Could you check a few things on this model? Use its own coordinates, in mm. A direction names the side the tool comes from. Coordinates: 2 decimals unless noted, no trailing zeros. Write each loop counter-clockwise with the first axis right and the second up, starting at its lowest first coordinate (ties: lowest second). Pieces come first, ordered by that corner, then holes.
```python
from build123d import *

# Parameters (mm, degrees)
SKETCH1_R               = 14.2875
SKETCH1_R_2             = 9.525
BOSS_EXTRUDE1_DEPTH     = 3.175
F_10_CLEARANCE_HOLE2_D  = 4.9784
F_10_CLEARANCE_HOLE3_D  = 4.9784
F_1_4_CLEARANCE_HOLE1_D = 6.5278


with BuildPart() as part:
    # Sketch1 → Boss-Extrude1 (new body)
    with BuildSketch(Plane.XY.offset(-14.194599474)):
        with BuildLine():
            Line((-11.403602879, 461.040918113), (18.881283072, 509.506866808))
            Line((18.881283072, 509.506866808), (22.784668372, 515.753589084))
            Line((22.784668372, 515.753589084), (19.342339301, 522.227668471))
            Line((19.342339301, 522.227668471), (12.014457551, 522.48356374))
            Line((12.014457551, 522.48356374), (8.11107225, 516.236841464))
            Line((8.11107225, 516.236841464), (-23.846467356, 536.206128526))
            Line((-23.846467356, 536.206128526), (10.759214603, 591.586796266))
            Line((10.759214603, 591.586796266), (24.22197813, 583.174327946))
            Line((24.22197813, 583.174327946), (51.141876753, 626.255171231))
            Line((51.141876753, 626.255171231), (112.462044501, 660.93728694))
            ThreePointArc((112.462044501, 660.93728694), (123.365099157, 699.702028841), (84.677956887, 710.877306848))
            Line((84.677956887, 710.877306848), (-5.401730059, 661.587538174))
            Line((-5.401730059, 661.587538174), (-69.615486106, 558.824047132))
            Line((-69.615486106, 558.824047132), (-54.307899735, 487.850498283))
            Line((-54.307899735, 487.850498283), (-11.403602879, 461.040918113))
        make_face()
        with Locations((16.14150623, 618.174698631)):
            Circle(SKETCH1_R, mode=Mode.SUBTRACT)
        with Locations((-22.373657227, 496.622766323)):
            Circle(SKETCH1_R_2, mode=Mode.SUBTRACT)
        with Locations((98.394472266, 685.809641802)):
            Circle(SKETCH1_R, mode=Mode.SUBTRACT)
    extrude(amount=BOSS_EXTRUDE1_DEPTH)

    # #10 Clearance Hole2 (through all)
    with Locations(Plane.XY.offset(-11.019599474)):
        with Locations((2.375342418, 502.336523103), (-47.122656873, 490.909009542), (-3.381611976, 652.837445435), (42.391784014, 624.235053148), (22.201860047, 591.924420685), (-23.571535943, 620.526812972), (-31.474844299, 535.981130963), (-63.785476762, 556.17105493), (-51.664768266, 503.670498499), (2.009121865, 589.566678183), (-30.301510599, 609.756602151)):
            Hole(F_10_CLEARANCE_HOLE2_D / 2)

    # #10 Clearance Hole3 (through all)
    with Locations(Plane.XY.offset(-11.019599474)):
        with Locations((111.013174745, 706.003787092), (122.192466334, 684.978597537), (109.573763855, 664.784452247), (85.775769786, 665.615496512), (74.596478197, 686.640686067), (87.215180677, 706.834831357)):
            Hole(F_10_CLEARANCE_HOLE3_D / 2)

    # 1/4 Clearance Hole1 (through all)
    with Locations(Plane.XY.offset(-11.019599474)):
        with Locations((15.456786622, 516.009484354)):
            Hole(F_1_4_CLEARANCE_HOLE1_D / 2)


solid = part.part
```
Item 1: Which directions (+Z, -Z, +X, -X, +Y, -Y) give clear straight access to the entire face, cutting with the end or side of a thin tool? Please do faces 1 (the flat face through (6, 607, -11.02)), 2 (the flat face through (-7.64, 526.08, -12.63)).
Item 2: Will this pin go through, and if not, where does the flat tip stop? pin 1 Ø1.5 at (y, z) = (490, -13) entering from +X.
Item 3: If I drill on line 1 along Y through (x, z) = (23, -13.95); line 2 along Y through (x, z) = (14.5, -13.45); line 3 along Y through (x, z) = (22.5, -13.25), over which ranges is the centre line in solid material (lowest first)?
Item 4: I want a section at A-A, the plane x = -40. List the corners of the cut face in (y, z) for me, then the cut area to 3 significant figures.
Item 5: I want a section at B-B, the plane z = -12.9. Count the separate pieces of the cut face and the enclosed holes in it, then the cut area to 3 significant figures.
Item 6: I want a section at C-C, the plane x = 60. List the corners of the cut face in (y, z) for me, then the cut area to 3 significant figures.
Item 7: If we mould it in two halves opening along X, with no side actions, what happens to faces 3 (the cylindrical face through (-46.58, 488.48, -12.63)), 4 (the flat face through (6, 607, -14.195)), 5 (the flat face through (-37.059, 610.925, -12.629))? For each: released by +X, released by -X, zero draft, split by the parting line, or undercut.
Taken from the geometry:
1. face 1: +Z, +X, -X, +Y, -Y
1. face 2: +Z, -Z
2. pin 1: stops at x = 7.16
3. line 1: y = 583.94 to 589.57, 594.28 to 605.64, 630.71 to 677.13
3. line 2: y = 502.5 to 512.89, 519.13 to 522.4, 589.25 to 603.98, 632.37 to 672.48
3. line 3: y = 515.3 to 516.29, 584.25 to 589.45, 594.4 to 605.38, 630.97 to 676.85
4. outline: (478.91, -14.19) - (606.22, -14.19) - (606.22, -11.02) - (478.91, -11.02) - close
4. area: 404 mm2
5. separate pieces: 1
5. enclosed holes: 21
5. area: 15,600 mm2
6. outline: (631.27, -14.19) - (697.37, -14.19) - (697.37, -11.02) - (631.27, -11.02) - close
6. area: 210 mm2
7. face 3: undercut
7. face 4: zero draft
7. face 5: released by -X
